Model file for the job. Use its own axes, mm. Face numbers are marked on the shaded views. A direction names the side the tool comes from. Give positions to 0.01 mm unless a question says otherwise; leave off trailing zeros. Loops run counter-clockwise (first coordinate to the right, second up) from the corner with the lowest first, then second, coordinate; pieces in that order, holes last. Notation, with made-up numbers: M 29,3 L 81,3 A14 cw 81,14 Z; hole C -37.5,-31.5 d9. An arc over 180 degrees is marked long. Use CSV: the item, a comma, the result in double quotes. Start each with the question number.
(1) Wall check: line 1 along Y through (x, z) = (0, 4.3); line 2 along Z through (x, y) = (-6, 4.75); line 3 along Y through (x, z) = (0, 2.9). Give the ranges that are in metal, low to high. Write a range as from..to.
(2) Flat gauge pins, fed straight in: P1, Ø1, axis at y = 1, z = 4.5, coming from the +X side; P2, Ø1, axis at y = 2.5, z = 5, coming from the -X side; P3, Ø2, axis at x = 5, y = -1, coming from the -Z side; P4, Ø3, axis at x = 0, y = 0, coming from the -Z side. Where does each tip first touch, or does it go through?
(3) Two-plate mould, pull along Y, no slides. Class the marked faces 1, 2, 3 and 4: pulls with the +Y half, pulls with the -Y half, needs draft (parallel to the pull), parting line crosses it, or undercut.
(4) Slice it at A-A on x = 0. List the corners of the cut face in (y, z).
(5) Tool access for the marked faces 5 and 6: list every direction of +Z, -Z, +X, -X, +Y, -Y with a clear straight run to the whole face (end or side of a thin tool).
(6) Slice it at C-C on z = 1. List the corners of the cut face in (x, y).
(7) Slice it at D-D on x = 5.75. List the corners of the cut face in (y, z), and give its area (3 significant figures).
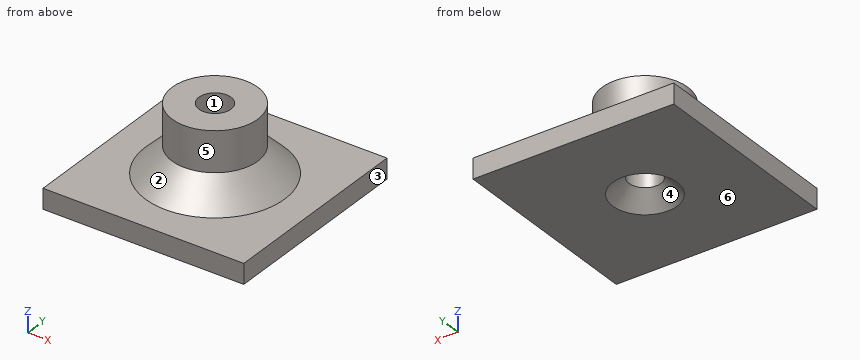
```python
from build123d import *

# Parameters (mm, degrees)
SKETCH_2_W        = 15
SKETCH_2_H        = 15
SKETCH_2_R        = 1.2
EXTRUDE_430_DEPTH = 1.5
SKETCH_3_R        = 3.2
SKETCH_3_R_2      = 1.2
EXTRUDE_671_DEPTH = 5
CHAMFER_1_SIZE    = 1.2
CHAMFER_2_SIZE    = 2


with BuildPart() as part:
    # Эскиз2 → Extrude 430 (new body)
    with BuildSketch(Plane.XY):
        Rectangle(SKETCH_2_W, SKETCH_2_H)
        Circle(SKETCH_2_R, mode=Mode.SUBTRACT)
    extrude(amount=EXTRUDE_430_DEPTH)

    # Эскиз3 → Extrude 671 (add)
    with BuildSketch(Plane.XY.offset(1.5)):
        with Locations(Location((0, 0, 0), (0, 0, 180))):
            Circle(SKETCH_3_R)
        Circle(SKETCH_3_R_2, mode=Mode.SUBTRACT)
    extrude(amount=EXTRUDE_671_DEPTH)

    # Фаска1
    chamfer_1_edges = [part.edges().sort_by_distance(p)[0] for p in [
        (-1.2, 0, 0),
    ]]
    chamfer(chamfer_1_edges, length=CHAMFER_1_SIZE)

    # Фаска2
    chamfer_2_edges = [part.edges().sort_by_distance(p)[0] for p in [
        (3.2, 0, 1.5),
    ]]
    chamfer(chamfer_2_edges, length=CHAMFER_2_SIZE)


solid = part.part
```
Reply:
1,line 1,"y = -3.2..-1.2, 1.2..3.2"
1,line 2,"z = 0..1.5"
1,line 3,"y = -3.8..-1.2, 1.2..3.8"
2,P1,"stops at x = 3.16"
2,P2,"stops at x = -2.5"
2,P3,"stops at z = 0"
2,P4,"stops at z = 0.9"
3,face 1,"undercut"
3,face 2,"parting line crosses it"
3,face 3,"needs draft"
3,face 4,"undercut"
4,outline,"M -7.5,0 L -2.4,0 L -1.2,1.2 L -1.2,6.5 L -3.2,6.5 L -3.2,3.5 L -5.2,1.5 L -7.5,1.5 Z; M 1.2,1.2 L 2.4,0 L 7.5,0 L 7.5,1.5 L 5.2,1.5 L 3.2,3.5 L 3.2,6.5 L 1.2,6.5 Z"
5,face 5,"+Z"
5,face 6,"-Z, +X, -X, +Y, -Y"
6,outline,"M -7.5,-7.5 L 7.5,-7.5 L 7.5,7.5 L -7.5,7.5 Z; hole C 0,0 d2.8"
7,outline,"M -7.5,0 L 7.5,0 L 7.5,1.5 L -7.5,1.5 Z"
7,area,"22.5 mm^2"
